Can you work these out from the model? Positions are in its coordinate system, mm. A direction names the side the tool comes from. Give positions to 0.01 mm unless a question says otherwise; leave off trailing zeros. Order: outer loops, then holes, each group sorted by start corner. A loop starts at its lowest first (then second) coordinate and runs counter-clockwise, first axis right, second up. Notation, with made-up numbers: (-6, 29.5) - (27, 29.5) arc R25 cw to (27, 60.5) - close; hole circle Ø9 at (-8.75, 85.25). An arc over 180 degrees is marked (long way). Return JSON: item names as keys, results as strings.
```python
from build123d import *

# Parameters (mm, degrees)
F0_W     = 78.858778
F0_H     = 70.800216
F1_DEPTH = 76.2
F2_W     = 22.448848
F2_H     = 35.400108
F3_DEPTH = 25.4
F5_W     = 34.536688
F5_H     = 33.673274
F6_DEPTH = 25.4


with BuildPart() as f1:
    # F0 (on Top) → F1 (new body)
    with BuildSketch(Plane.XY):
        Rectangle(F0_W, F0_H)
        Polygon((0, 72.239242), (-39.429389, 35.400108), (39.429389, 35.400108), align=None)
    extrude(amount=F1_DEPTH)

    # F2 (on face) → F3 (cut)
    with BuildSketch(Plane.XY.offset(76.2)):
        with Locations((-14.390288, -17.700054)):
            Rectangle(F2_W, F2_H)
    extrude(amount=-F3_DEPTH, mode=Mode.SUBTRACT)

    # F5 (on face) → F6 (cut)
    with BuildSketch(Plane.XY.offset(76.2)):
        with Locations((5.468308, 25.758615)):
            Rectangle(F5_W, F5_H)
    extrude(amount=-F6_DEPTH, mode=Mode.SUBTRACT)


solid = f1.part
```
1. If I drill on L1, parallel to X at y = -21.5, z = 53; L2, parallel to Z at x = 15, y = 27.5; L3, parallel to X at y = 62.5, z = 64, over which ranges is the centre line in solid material (lowest first)? Write a range as [from, to].
Checks:
{"L1": "[-39.43, -25.61], [-3.17, 39.43]", "L2": "[0, 50.8]", "L3": "[-10.42, 10.42]"}
2. Suppose I cut it at D-D (z = 27.5). List the corners of the cut face in (x, y) for me, plus the area to 3 significant figures.
Checks:
{"outline": "(-39.43, -35.4) - (39.43, -35.4) - (39.43, 35.4) - (0, 72.24) - (-39.43, 35.4) - close", "area": "7,040 mm^2"}
3. For pin 1 Ø17 at (x, y) = (4.5, 22) entering from +Z; pin 2 Ø2 at (y, z) = (53.5, 36) entering from -X; pin 3 Ø4 at (x, z) = (-31, 30) entering from +Y, each with a flat end and sliding along its axis, tell me the tip position at first contact or that it passes through.
Checks:
{"pin 1": "z = 50.8", "pin 2": "x = -21.13", "pin 3": "y = 45.14"}
4. Suppose I cut it at B-B (z = 63.5). List the corners of the cut face in (x, y) for me.
Checks:
{"outline": "(-39.43, -35.4) - (-25.61, -35.4) - (-25.61, 0) - (-3.17, 0) - (-3.17, -35.4) - (39.43, -35.4) - (39.43, 35.4) - (0, 72.24) - (-39.43, 35.4) - close; hole (-11.8, 8.92) - (22.74, 8.92) - (22.74, 42.6) - (-11.8, 42.6) - close"}
5. Thinking about a two-plate mould opening in Y: for faces 4 (the face through (-15, 0, 64)), 5 (the face through (5, 42.595, 64)), 6 (the face through (-1, 7, 76.2)), which applies, +Y half, -Y half, draft (parallel to the pull), parting line (faces both ways), or undercut?
Checks:
{"face 4": "-Y half", "face 5": "undercut", "face 6": "draft"}
6. On a 3-axis mill with a long thin cutter (end or side, diameter ignored), from which of +Z, -Z, +X, -X, +Y, -Y can I reach the whole of each face in a straight line? I mean faces 1 (the face through (5, 8.922, 64)), 2 (the face through (-19.439, 54.078, 37.567)), 3 (the face through (-3.166, -18, 64)). Say none if no direction works.
Checks:
{"face 1": "+Z", "face 2": "+Z, -Z, -X, +Y", "face 3": "+Z, -Y"}
7. Suppose I cut it at C-C (x = 19.5). List the corners of the cut face in (y, z) for me.
Checks:
{"outline": "(-35.4, 0) - (54.02, 0) - (54.02, 76.2) - (42.6, 76.2) - (42.6, 50.8) - (8.92, 50.8) - (8.92, 76.2) - (-35.4, 76.2) - close"}
8. Suppose I cut it at A-A (y = -12.5). List the corners of the cut face in (x, z) for me.
Checks:
{"outline": "(-39.43, 0) - (39.43, 0) - (39.43, 76.2) - (-3.17, 76.2) - (-3.17, 50.8) - (-25.61, 50.8) - (-25.61, 76.2) - (-39.43, 76.2) - close"}
